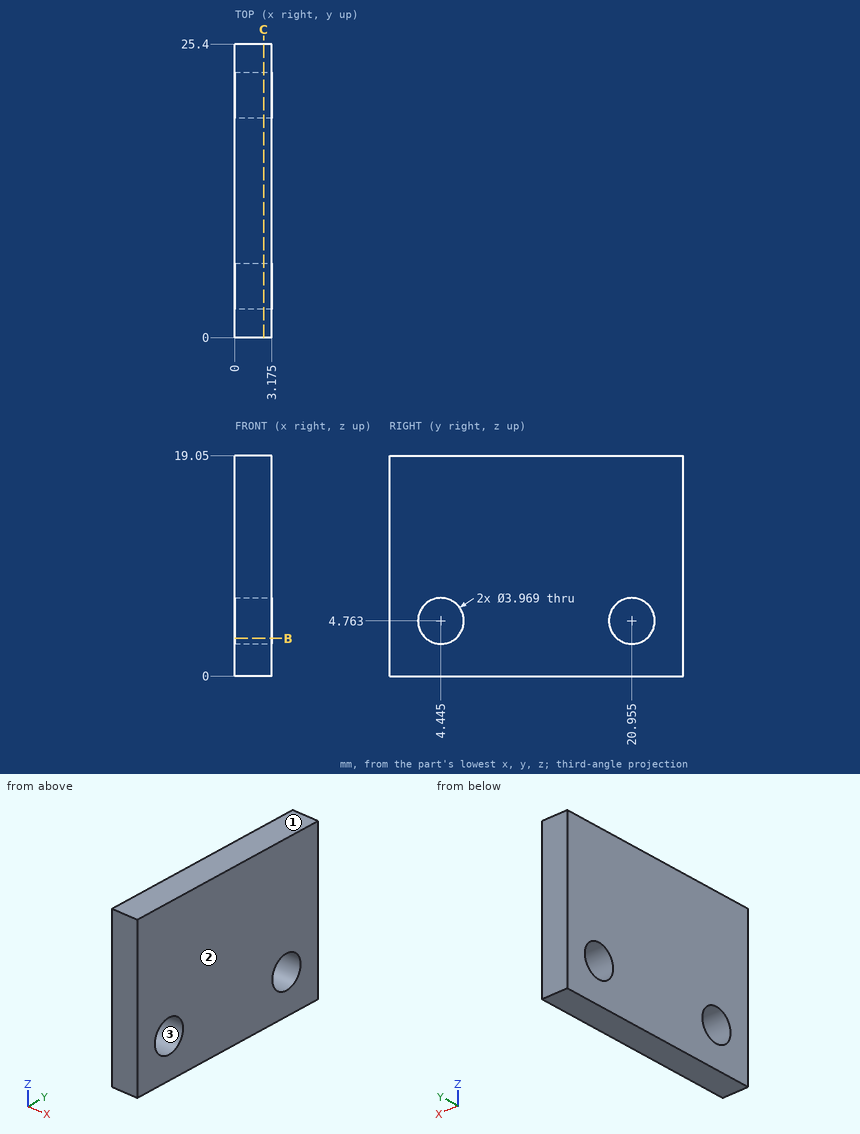
Could you check a few things on this drawing? It's one solid part, dimensions in mm from its lowest x, y, z. Coordinates: 2 decimals unless noted, no trailing zeros. Write each loop counter-clockwise with the first axis right and the second up, starting at its lowest first coordinate (ties: lowest second). Pieces come first, ordered by that corner, then holes. Notation, with made-up numbers: (12.5, 14.25) - (52.5, 14.25) arc R29 ccw to (52.5, 51.25) - close; hole circle Ø11 at (27.5, -9). An arc over 180 degrees is marked (long way). Use one line per item in the form item = value.
1) Thinking about a two-plate mould opening in Z: for the marked faces 1, 2 and 3, which applies, released by +Z, released by -Z, zero draft, split by the parting line, or undercut?
Solved:
face_1 = released by +Z
face_2 = zero draft
face_3 = undercut
2) Suppose I cut it at C-C, the plane x = 2.5. Give the number of separate pieces and of enclosed holes in the cut face, plus the area to 3 significant figures.
Solved:
separate_pieces = 1
enclosed_holes = 2
area = 459 mm2
3) Suppose I cut it at B-B, the plane z = 3.25. Write out the boundary of the cut face in (x, y) (1 decimal).
Solved:
outline = (0, 0) - (3.2, 0) - (3.2, 3.2) - (0, 3.2) - close; (0, 5.7) - (3.2, 5.7) - (3.2, 19.7) - (0, 19.7) - close; (0, 22.2) - (3.2, 22.2) - (3.2, 25.4) - (0, 25.4) - close
4) I need wall thicknesses on line 1 (Y direction, x = 2.1, z = 4.75); line 2 (Y direction, x = 1.3, z = 5.75) (1 decimal); line 3 (Z direction, x = 2.4, y = 21). Which ranges of each line are inside material? Lowest first, please.
Solved:
line_1 = 0 to 2.46, 6.43 to 18.97, 22.94 to 25.4
line_2 = 0 to 2.7, 6.2 to 19.2, 22.7 to 25.4
line_3 = 0 to 2.78, 6.75 to 19.05
